Verification items for the finished model (mm, model axes). Round coordinates to 2 decimals unless told otherwise and drop trailing zeros. Write each loop counter-clockwise with the first axis right and the second up, starting at its lowest first coordinate (ties: lowest second). Pieces come first, ordered by that corner, then holes. Notation, with made-up numbers: M 17.25,41 L 46.25,41 A18 ccw 46.25,46 Z; hole C -19,13 d3. An arc over 180 degrees is marked long. Answer in a Markdown table with one row per item. Add a question column.
1. Go/stop test with flat-tipped pins: pin 1 Ø1.5 at (y, z) = (2.5, -247.5) entering from -X; pin 2 Ø2.5 at (y, z) = (1.5, -198.5) entering from -X; pin 3 Ø1.6 at (x, y) = (328.5, 1.5) entering from +Z. Record where each tip stops, or that it passes through.
2. Sectioned sample at A-A on y = 5. Record the cut outline in (x, z).
3. Sectioned sample at B-B on x = 297.5. Record the cut outline in (y, z) (3 decimals), plus the area to 3 significant figures.
4. Material ranges on probe 1 along Z at (x, y) = (321.5, 3.25); probe 2 along Z at (x, y) = (359, 5.25); probe 3 along X at (y, z) = (2.75, -43), recorded low to high.
```python
from build123d import *

# Parameters (mm, degrees)
BOSS_EXTRUDE1_DEPTH = 6.35
CUT_EXTRUDE2_DEPTH  = 3.175
FILLET1_R           = 5.08


with BuildPart() as part:
    # Sketch1 → Boss-Extrude1 (new body)
    with BuildSketch(Plane(origin=(0, 0, 0), x_dir=(1, 0, 0), z_dir=(0, 1, 0))):
        Polygon((172.72, 12.7), (172.72, 273.759815483), (228.6, 370.54681461), (435.202954744, 12.7), align=None)
        Polygon((185.42, 25.4), (413.205909488, 25.4), (228.6, 345.14681461), (185.42, 270.356860739), align=None, mode=Mode.SUBTRACT)
        Polygon((185.42, 25.4), (185.42, 270.356860739), (228.6, 345.14681461), (413.205909488, 25.4), align=None)
    extrude(amount=BOSS_EXTRUDE1_DEPTH)

    # Sketch1_3 → Cut-Extrude2 (cut)
    with BuildSketch(Plane(origin=(0, 0, 0), x_dir=(1, 0, 0), z_dir=(0, 1, 0))):
        Polygon((172.72, 12.7), (172.72, 273.759815483), (228.6, 370.54681461), (435.202954744, 12.7), align=None)
        Polygon((185.42, 25.4), (413.205909488, 25.4), (228.6, 345.14681461), (185.42, 270.356860739), align=None, mode=Mode.SUBTRACT)
    extrude(amount=CUT_EXTRUDE2_DEPTH, mode=Mode.SUBTRACT)

    # Fillet1
    fillet1_edges = [part.edges().sort_by_distance(p)[0] for p in [
        (172.72, 4.7625, -273.759815483),
        (228.6, 4.7625, -370.54681461),
        (435.202954744, 4.7625, -12.7),
        (172.72, 4.7625, -12.7),
    ]]
    fillet(fillet1_edges, radius=FILLET1_R)


solid = part.part
```
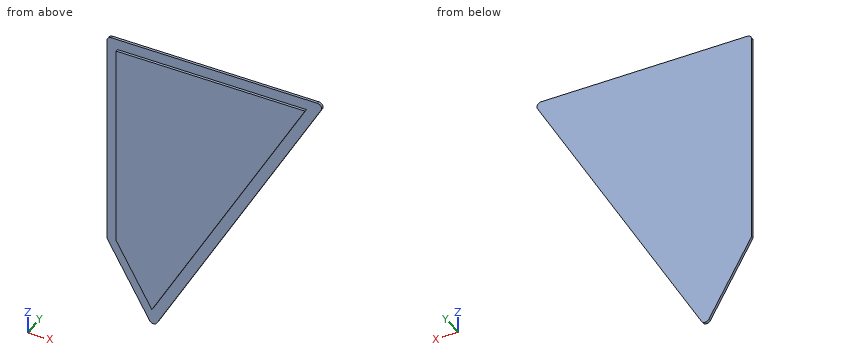
Geometry check:
| question | item | result |
|---|---|---|
| 1 | pin 1 | stops at x = 172.72 |
| 1 | pin 2 | stops at x = 185.42 |
| 1 | pin 3 | stops at z = -25.4 |
| 2 | outline | M 172.72,-272.4 A5.08 ccw 173.4,-274.94 L 224.2,-362.93 A5.08 ccw 233,-362.93 L 430.8,-20.32 A5.08 ccw 426.4,-12.7 L 177.8,-12.7 A5.08 ccw 172.72,-17.78 Z |
| 3 | outline | M 0,-225.809 L 3.175,-225.809 L 3.175,-251.209 L 6.35,-251.209 L 6.35,-12.7 L 3.175,-12.7 L 3.175,-25.4 L 0,-25.4 Z |
| 3 | area | 1,390 mm2 |
| 4 | probe 1 | z = -209.64 to -12.7 |
| 4 | probe 2 | z = -144.69 to -12.7 |
| 4 | probe 3 | x = 185.42 to 403.04 |
